The model under review builds one solid part; all positions refer to its coordinate system, in mm. Give positions to 0.01 mm unless a question says otherwise; leave off trailing zeros. Order: outer loops, then holes, each group sorted by start corner. A loop starts at its lowest first (then second) coordinate and runs counter-clockwise, first axis right, second up.
```python
from build123d import *

# Parameters (mm, degrees)
SKETCH1_W           = 220
SKETCH1_H           = 110
BOSS_EXTRUDE1_DEPTH = 20
SKETCH2_R           = 12.5
SKETCH2_R_2         = 7.6
CUT_EXTRUDE1_DEPTH  = 15
CHAMFER1_SIZE       = 1
FILLET1_R           = 1
SKETCH4_R           = 11.5
CUT_EXTRUDE2_DEPTH  = 5
FILLET2_R           = 10


with BuildPart() as part:
    # Sketch1 → Boss-Extrude1 (new body)
    with BuildSketch(Plane(origin=(0, 0, 0), x_dir=(1, 0, 0), z_dir=(0, 1, 0))):
        with Locations((110, 55)):
            Rectangle(SKETCH1_W, SKETCH1_H)
    extrude(amount=BOSS_EXTRUDE1_DEPTH)

    # Sketch2 → Cut-Extrude1 (cut)
    with BuildSketch(Plane(origin=(0, 20, 0), x_dir=(1, 0, 0), z_dir=(0, 1, 0))):
        with Locations(Location((17.5, 45, 0), (0, 0, 270))):
            Circle(SKETCH2_R)
        with Locations(Location((202.5, 45, 0), (0, 0, 90))):
            Circle(SKETCH2_R)
        with Locations(Location((110, 15, 0), (0, 0, 270))):
            Circle(SKETCH2_R_2)
    extrude(amount=-CUT_EXTRUDE1_DEPTH, mode=Mode.SUBTRACT)

    # Chamfer1
    chamfer1_edges = [part.edges().sort_by_distance(p)[0] for p in [
        (17.5, 20, -57.5),
        (202.5, 20, -32.5),
    ]]
    chamfer(chamfer1_edges, length=CHAMFER1_SIZE)

    # Fillet1
    fillet1_edges = [part.edges().sort_by_distance(p)[0] for p in [
        (202.5, 19, -32.5),
        (17.5, 19, -57.5),
    ]]
    fillet(fillet1_edges, radius=FILLET1_R)

    # Sketch4 → Cut-Extrude2 (cut)
    with BuildSketch(Plane(origin=(0, 20, 0), x_dir=(1, 0, 0), z_dir=(0, 1, 0))):
        with Locations(Location((110, 15, 0), (0, 0, 270))):
            Circle(SKETCH4_R)
    extrude(amount=-CUT_EXTRUDE2_DEPTH, mode=Mode.SUBTRACT)

    # Fillet2
    fillet2_edges = [part.edges().sort_by_distance(p)[0] for p in [
        (0, 10, -110),
        (220, 10, -110),
        (220, 10, 0),
        (0, 10, 0),
    ]]
    fillet(fillet2_edges, radius=FILLET2_R)


solid = part.part
```
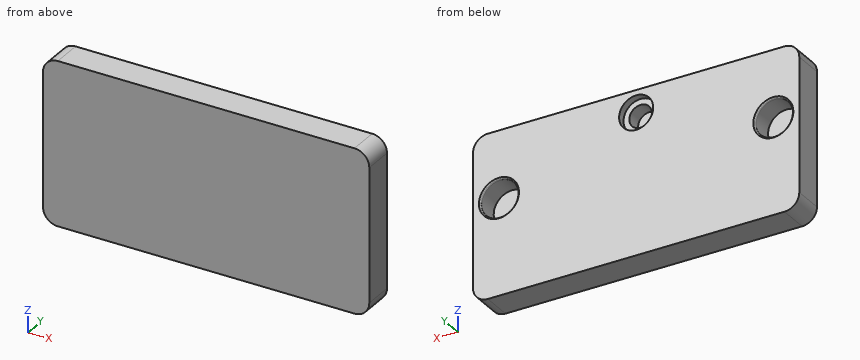
1. To check wall thickness, follow line 1 (X direction, y = 8.5, z = -45); line 2 (X direction, y = 8.75, z = -15); line 3 (X direction, y = 18.25, z = -54). State the ranges of each line that lie inside material, in increasing order.
2. Take a section at B-B (x = 110). Write out the cut boundary in (y, z), and give its area (3 significant figures).
3. Take a section at C-C (z = -15). Write out the cut boundary in (x, y).
4. Take a section at A-A (y = 12.25). Write out the cut boundary in (x, z), and give its area (3 significant figures).
5. Insertion check: pin 1 (15 mm diameter, centred on x = 17.5, z = -45, fed in from +Y); pin 2 (16.5 mm diameter, centred on x = 109, z = -18, fed in from +Y). Each pin has a flat end and moves straight along its axis. Give the tip position at first contact, or say it passes through.
Answer:
1. line 1: x = 0 to 5, 30 to 190, 215 to 220
1. line 2: x = 0 to 102.4, 117.6 to 220
1. line 3: x = 0 to 8.83, 26.17 to 193.83, 211.17 to 220
2. outline: (0, -110) - (20, -110) - (20, -26.5) - (15, -26.5) - (15, -22.6) - (5, -22.6) - (5, -7.4) - (15, -7.4) - (15, -3.5) - (20, -3.5) - (20, 0) - (0, 0) - close
2. area: 1,930 mm2
3. outline: (0, 0) - (220, 0) - (220, 20) - (121.5, 20) - (121.5, 15) - (117.6, 15) - (117.6, 5) - (102.4, 5) - (102.4, 15) - (98.5, 15) - (98.5, 20) - (0, 20) - close
4. outline: (0, -100) arc R10 ccw to (10, -110) - (210, -110) arc R10 ccw to (220, -100) - (220, -10) arc R10 ccw to (210, 0) - (10, 0) arc R10 ccw to (0, -10) - close; hole circle Ø25 at (17.5, -45); hole circle Ø15.2 at (110, -15); hole circle Ø25 at (202.5, -45)
4. area: 23,000 mm2
5. pin 1: stops at y = 5
5. pin 2: stops at y = 15
